Geometry: see drawing. Coordinates: mm, zero at the bounding-box minimum. Coordinates: 2 decimals unless noted, no trailing zeros. Order: outer loops, then holes, each group sorted by start corner. A loop starts at its lowest first (then second) coordinate and runs counter-clockwise, first axis right, second up.
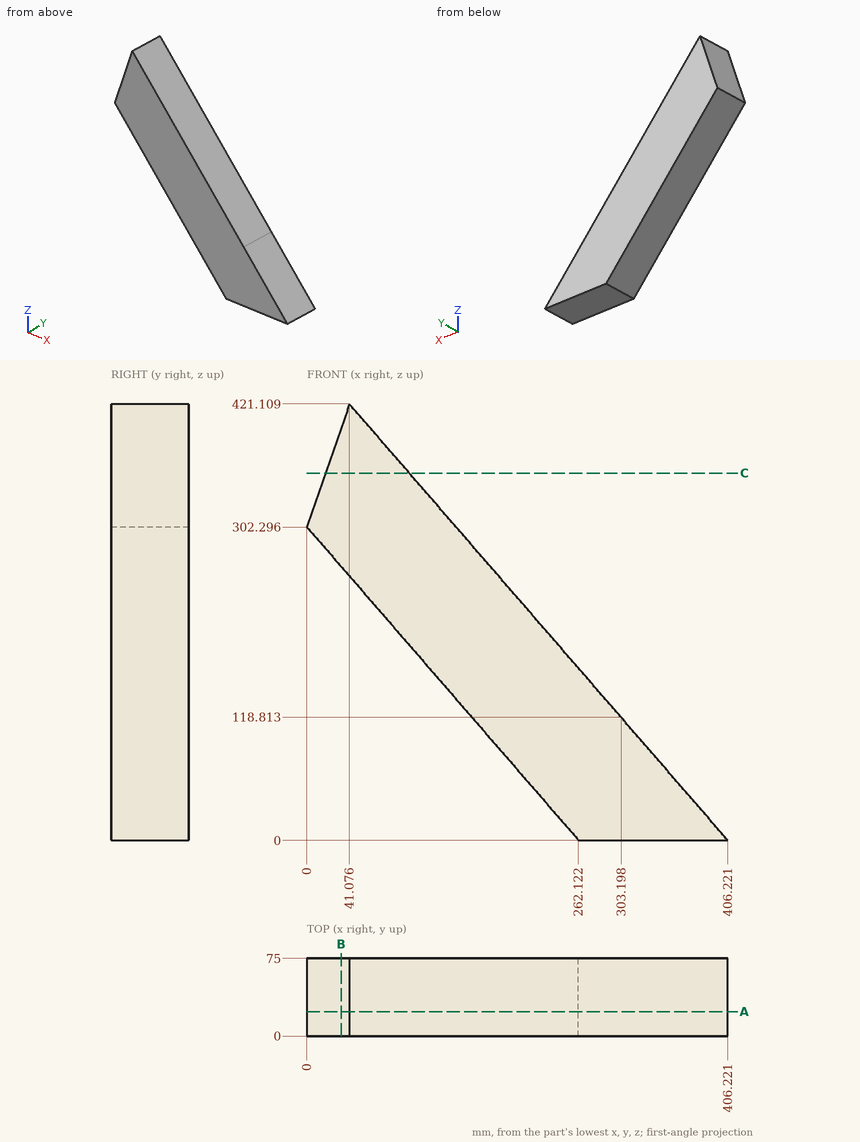
Item 1: Pin query (flat end, axial travel): pin 1 Ø8 at (y, z) = (57.5, 284.5) entering from +X; pin 2 Ø4 at (y, z) = (43, 343) entering from -X; pin 3 Ø4 at (x, y) = (121.5, 44.5) entering from +Z (1 decimal). Return the tip coordinate at first contact, or that it passes through.
Response values:
pin 1: stops at x = 163
pin 2: stops at x = 13.38
pin 3: stops at z = 330.7
Item 2: Ray query, probe 1 along Z at (x, y) = (323, 62.5) (1 decimal); probe 2 along Z at (x, y) = (197.5, 63) (1 decimal); probe 3 along X at (y, z) = (44, 321) (1 decimal). Return the intervals inside material, ascending.
Response values:
probe 1: z = 0 to 96
probe 2: z = 74.5 to 240.7
probe 3: x = 6.5 to 127.9
Item 3: Cut plane A-A on y = 23.5. Return loops of the section in (x, z) (1 decimal).
Response values:
outline: (0, 302.3) - (262.1, 0) - (406.2, 0) - (41.1, 421.1) - close
Item 4: Cut plane C-C on z = 354.5. Return loops of the section in (x, y).
Response values:
outline: (18.05, 0) - (98.83, 0) - (98.83, 75) - (18.05, 75) - close
Item 5: Cut plane B-B on x = 33. Return loops of the section in (y, z), then the cut area to 3 significant figures.
Response values:
outline: (0, 264.24) - (75, 264.24) - (75, 397.75) - (0, 397.75) - close
area: 10,000 mm2
